Check sheet for the modelled part. Datum: model origin and axes. Units: mm. Face numbers are marked on the shaded views. A direction names the side the tool comes from. Coordinates: 2 decimals unless noted, no trailing zeros. Order: outer loops, then holes, each group sorted by start corner. A loop starts at its lowest first (then second) coordinate and runs counter-clockwise, first axis right, second up. Notation, with made-up numbers: (35, 35.5) -> (93, 35.5) arc R20 cw to (93, 73.5) -> close; hole circle Ø9 at (42.25, 15.25). An arc over 180 degrees is marked (long way). Put each result on its own line as item: value. Start each with the question number.
```python
from build123d import *

# Parameters (mm, degrees)
BOSS_EXTRU_1_DEPTH      = 12
ENL_V_MAT_EXTRU_1_DEPTH = 4
ESQUISSE3_R             = 8
ENL_V_MAT_EXTRU_2_DEPTH = 41.853396432
ESQUISSE4_W             = 50
ESQUISSE4_H             = 12
BOSS_EXTRU_2_DEPTH      = 25
ENL_V_MAT_EXTRU_3_DEPTH = 66.383484153
ESQUISSE7_W             = 50
ESQUISSE7_H             = 20
BOSS_EXTRU_3_DEPTH      = 30
ESQUISSE9_W             = 50
ESQUISSE9_H             = 12
BOSS_EXTRU_4_DEPTH      = 6
ESQUISSE10_R            = 5
ENL_V_MAT_EXTRU_4_DEPTH = 95.212525707
ESQUISSE11_R            = 7.5
ENL_V_MAT_EXTRU_5_DEPTH = 84.671978613


with BuildPart() as part:
    # Esquisse1 → Boss.-Extru.1 (new body)
    with BuildSketch(Plane(origin=(0, 0, 0), x_dir=(1, 0, 0), z_dir=(0, 1, 0))):
        with BuildLine():
            Line((-25, 0), (-25, 30))
            Line((-25, 30), (25, 30))
            Line((25, 30), (25, 0))
            ThreePointArc((25, 0), (0, -25), (-25, 0))
        make_face()
    extrude(amount=-BOSS_EXTRU_1_DEPTH)

    # Esquisse2 → Enlèv. mat.-Extru.1 (cut)
    with BuildSketch(Plane(origin=(0, 0, 0), x_dir=(1, 0, 0), z_dir=(0, 1, 0))):
        with BuildLine():
            Line((-22.5, 30), (22.5, 30))
            Line((22.5, 30), (22.5, -10.897247359))
            ThreePointArc((22.5, -10.897247359), (0, -25), (-22.5, -10.897247359))
            Line((-22.5, -10.897247359), (-22.5, 30))
        make_face()
    extrude(amount=-ENL_V_MAT_EXTRU_1_DEPTH, mode=Mode.SUBTRACT)

    # Esquisse3 → Enlèv. mat.-Extru.2 (cut, through all)
    with BuildSketch(Plane.XZ.offset(12)):
        with Locations(Location((0, 0, 0), (0, 0, 270))):
            Circle(ESQUISSE3_R)
    extrude(amount=-ENL_V_MAT_EXTRU_2_DEPTH, mode=Mode.SUBTRACT)

    # Esquisse4 → Boss.-Extru.2 (add)
    with BuildSketch(Plane(origin=(0, 0, 0), x_dir=(1, 0, 0), z_dir=(0, 1, 0))):
        with Locations((0, 36)):
            Rectangle(ESQUISSE4_W, ESQUISSE4_H)
    extrude(amount=-BOSS_EXTRU_2_DEPTH)

    # Esquisse5 → Enlèv. mat.-Extru.3 (cut, through all)
    with BuildSketch(Plane.XY.offset(-30)):
        with BuildLine():
            Line((12.834819399, -25), (-12.834819399, -25))
            ThreePointArc((-12.834819399, -25), (0, -12.165180601), (12.834819399, -25))
        make_face()
    extrude(amount=-ENL_V_MAT_EXTRU_3_DEPTH, mode=Mode.SUBTRACT)

    # Esquisse7 → Boss.-Extru.3 (add)
    with BuildSketch(Plane(origin=(0, 0, 0), x_dir=(1, 0, 0), z_dir=(0, 1, 0))):
        with Locations((0, 52)):
            Rectangle(ESQUISSE7_W, ESQUISSE7_H)
    extrude(amount=-BOSS_EXTRU_3_DEPTH)

    # Esquisse9 → Boss.-Extru.4 (add)
    with BuildSketch(Plane(origin=(0, 0, 0), x_dir=(1, 0, 0), z_dir=(0, 1, 0))):
        with Locations((0, 68)):
            Rectangle(ESQUISSE9_W, ESQUISSE9_H)
    extrude(amount=-BOSS_EXTRU_4_DEPTH)

    # Esquisse10 → Enlèv. mat.-Extru.4 (cut, through all)
    with BuildSketch(Plane(origin=(25, 0, 0), x_dir=(0, 0, -1), z_dir=(1, 0, 0))):
        with Locations((45, -12)):
            Circle(ESQUISSE10_R)
    extrude(amount=-ENL_V_MAT_EXTRU_4_DEPTH, mode=Mode.SUBTRACT)

    # Esquisse11 → Enlèv. mat.-Extru.5 (cut, through all)
    with BuildSketch(Plane.XZ.offset(30)):
        with Locations(Location((0, -52, 0), (0, 0, 270))):
            Circle(ESQUISSE11_R)
    extrude(amount=-ENL_V_MAT_EXTRU_5_DEPTH, mode=Mode.SUBTRACT)


solid = part.part
```
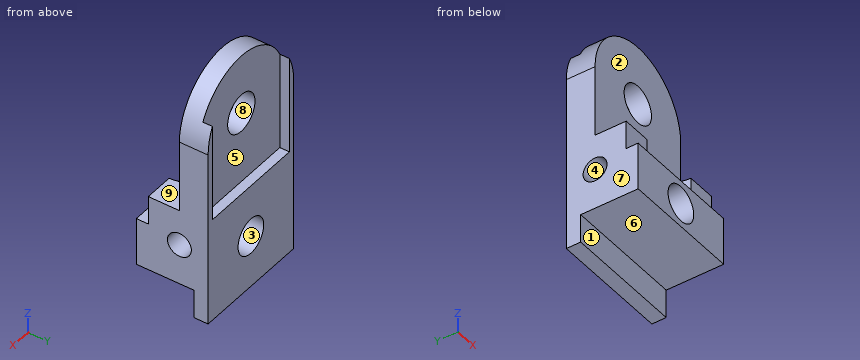
1) Scan lines: line 1 along Z through (x, y) = (0, -20); line 2 along X through (y, z) = (-14.5, -52.5); line 3 along Z through (x, y) = (0, -15.5). Record each from-to range of solid material in increasing order. Write a range as [from, to].
2) Mould release check, pull along Z, two halves, no side actions. Record for the marked faces 6, 7, 8 and 9: +Z half, -Z half, draft (parallel to the pull), parting line (faces both ways), or undercut.
3) Sectioned sample at A-A (z = -52). Record the boundary of the cut face in (x, y), plus the area to 3 significant figures.
4) Sectioned sample at B-B (y = -15). Record the boundary of the cut face in (x, z).
5) Gauge pin test, flat ends, axial feed: pin 1 (12 mm diameter, centred on x = 11.5, y = -6.5, fed in from -Z); pin 2 (5 mm diameter, centred on x = -8, y = -19.5, fed in from -Z); pin 3 (9.5 mm diameter, centred on x = 4, z = -67.5, fed in from -Y); pin 4 (1.2 mm diameter, centred on x = -9.5, y = -1.5, fed in from +Z). Record the tip position at first contact, or that the pin passes through.
6) Sectioned sample at C-C (x = 5.5). Record the boundary of the cut face in (y, z).
7) Access from +Z, -Z, +X, -X, +Y, -Y to the whole of each face (thin tool, end or side, straight path). Record for the marked faces 1, 2, 3, 4 and 5.
8) Sectioned sample at D-D (y = -24). Record the boundary of the cut face in (x, z), plus the area to 3 significant figures.
Entries:
1. line 1: z = [-62, -59.5], [-44.5, -42]
1. line 2: x = [-25, -7.48], [7.48, 25]
1. line 3: z = [-62, -59.5]
2. face 6: -Z half
2. face 7: draft
2. face 8: undercut
2. face 9: +Z half
3. outline: (-25, -30) -> (-7.5, -30) -> (-7.5, 0) -> (-25, 0) -> close; (7.5, -30) -> (25, -30) -> (25, 0) -> (7.5, 0) -> close
3. area: 1,050 mm2
4. outline: (-25, -62) -> (25, -62) -> (25, -49) -> (6.87, -49) arc R7.5 cw (long way) to (-6.87, -49) -> (-25, -49) -> close; (-25, -41) -> (-8.05, -41) -> (-8.05, -30) -> (-25, -30) -> close; (8.05, -41) -> (25, -41) -> (25, -30) -> (8.05, -30) -> close
5. pin 1: stops at z = -74
5. pin 2: stops at z = -62
5. pin 3: stops at y = -6
5. pin 4: stops at z = -30
6. outline: (-30, -62) -> (-6, -62) -> (-6, -74) -> (0, -74) -> (0, -57.1) -> (-30, -57.1) -> close; (-30, -46.9) -> (-16.62, -46.9) arc R5 cw to (-16, -42) -> (-30, -42) -> close; (-13.4, -40.2) arc R5 cw to (-7.38, -46.9) -> (0, -46.9) -> (0, -30) -> (-4, -30) -> (-4, -5.81) -> (-12, -5.81) -> (-12, -30) -> (-13.4, -30) -> close; (-12, 5.81) -> (-4, 5.81) -> (-4, 24.39) -> (-12, 24.39) -> close
7. face 1: -Z, +X, -X, -Y
7. face 2: +Z, +X, -X, -Y
7. face 3: +Y, -Y
7. face 4: +X, -X
7. face 5: +Z, +Y
8. outline: (-25, -62) -> (25, -62) -> (25, -30) -> (12.8, -30) -> (12.8, -42) -> (-12.8, -42) -> (-12.8, -30) -> (-25, -30) -> close; hole circle Ø15 at (0, -52)
8. area: 1,120 mm2
